from build123d import *

# Parameters (mm, degrees)
SKETCH_1_W               = 55
SKETCH_1_H               = 55
EXTRUDE_1_DEPTH          = 4
FILLET_1_R               = 3.5
SKETCH_2_R               = 13.15
CUT_EXTRUDE_1_DEPTH      = 4
SKETCH_3_R               = 2.1
CUT_EXTRUDE_2_DEPTH      = 4
PATTERN_CIRCULAR_1_COUNT = 4
CUT_EXTRUDE_3_DEPTH      = 4
PATTERN_CIRCULAR_2_COUNT = 4


with BuildPart() as part:
    # 草图1 → 凸台-拉伸1 (new body)
    with BuildSketch(Plane(origin=(0, 0, 0), x_dir=(1, 0, 0), z_dir=(0, 1, 0))):
        Rectangle(SKETCH_1_W, SKETCH_1_H)
    extrude(amount=EXTRUDE_1_DEPTH)

    # 圆角1
    fillet_1_edges = [part.edges().sort_by_distance(p)[0] for p in [
        (27.5, 2, 27.5),
        (-27.5, 2, 27.5),
        (-27.5, 2, -27.5),
        (27.5, 2, -27.5),
    ]]
    fillet(fillet_1_edges, radius=FILLET_1_R)

    # 草图2 → 切除-拉伸1 (cut)
    with BuildSketch(Plane(origin=(0, 4, 0), x_dir=(1, 0, 0), z_dir=(0, 1, 0))):
        with Locations(Location((0, 0, 0), (0, 0, 270))):
            Circle(SKETCH_2_R)
    extrude(amount=-CUT_EXTRUDE_1_DEPTH, mode=Mode.SUBTRACT)

    # 草图3 → 切除-拉伸2 (cut)
    with BuildSketch(Plane(origin=(0, 4, 0), x_dir=(1, 0, 0), z_dir=(0, 1, 0))):
        with Locations(Location((0, 17.5, 0), (0, 0, 270))):
            Circle(SKETCH_3_R)
    cut_extrude_2 = extrude(amount=-CUT_EXTRUDE_2_DEPTH, mode=Mode.SUBTRACT)

    # 阵列(圆周)1: 切除-拉伸2 ×4 about axis
    pattern_circular_1_axis = Axis((0, 0, 0), (0, 1, 0))
    for i in range(1, PATTERN_CIRCULAR_1_COUNT):
        add(cut_extrude_2.rotate(pattern_circular_1_axis, i * 360 / PATTERN_CIRCULAR_1_COUNT), mode=Mode.SUBTRACT)

    # 草图4 → 切除-拉伸3 (cut)
    with BuildSketch(Plane(origin=(0, 4, 0), x_dir=(1, 0, 0), z_dir=(0, 1, 0))):
        with BuildLine():
            ThreePointArc((-21.9, 24), (-25.48492424, 25.48492424), (-24, 21.9))
            Line((-24, 21.9), (-24, 24))
            Line((-24, 24), (-21.9, 24))
        make_face()
        with BuildLine():
            Line((-24, 24), (-24, 21.9))
            ThreePointArc((-24, 21.9), (-22.51507576, 22.51507576), (-21.9, 24))
            Line((-21.9, 24), (-24, 24))
        make_face()
    cut_extrude_3 = extrude(amount=-CUT_EXTRUDE_3_DEPTH, mode=Mode.SUBTRACT)

    # 阵列(圆周)2: 切除-拉伸3 ×4 about axis
    pattern_circular_2_axis = Axis((0, 0, 0), (0, 1, 0))
    for i in range(1, PATTERN_CIRCULAR_2_COUNT):
        add(cut_extrude_3.rotate(pattern_circular_2_axis, i * 360 / PATTERN_CIRCULAR_2_COUNT), mode=Mode.SUBTRACT)


solid = part.part
Check sheet for the modelled part. Datum: model origin and axes. Units: mm. Round coordinates to 2 decimals unless told otherwise and drop trailing zeros. Order: outer loops, then holes, each group sorted by start corner. A loop starts at its lowest first (then second) coordinate and runs counter-clockwise, first axis right, second up.
Q1. Cross-section at C-C, the plane y = 2.8. Give the number of separate pieces and of enclosed holes in the cut face, plus the area to 3 significant figures.
Filled sheet:
separate pieces: 1
enclosed holes: 9
area: 2,360 mm2
Q2. Scan lines: L1, parallel to X at y = 1.3, z = -17.5; L2, parallel to Z at x = 22.5, y = 0.35; L3, parallel to Z at x = 23, y = 0.8. Record each from-to range of solid material in increasing order.
Filled sheet:
L1: x = -27.5 to -2.1, 2.1 to 27.5
L2: z = -27.5 to -25.47, -22.53 to 22.53, 25.47 to 27.5
L3: z = -27.5 to -25.85, -22.15 to 22.15, 25.85 to 27.5
Q3. Cross-section at D-D, the plane x = 0. Enter the section's corners in (y, z), plus the area to 3 significant figures.
Filled sheet:
outline: (0, -27.5) - (4, -27.5) - (4, -19.6) - (0, -19.6) - close; (0, -15.4) - (4, -15.4) - (4, -13.15) - (0, -13.15) - close; (0, 13.15) - (4, 13.15) - (4, 15.4) - (0, 15.4) - close; (0, 19.6) - (4, 19.6) - (4, 27.5) - (0, 27.5) - close
area: 81.2 mm2
Q4. Cross-section at B-B, the plane x = -17.5. Enter the section's corners in (y, z).
Filled sheet:
outline: (0, -27.5) - (4, -27.5) - (4, -2.1) - (0, -2.1) - close; (0, 2.1) - (4, 2.1) - (4, 27.5) - (0, 27.5) - close
Q5. Draft check along Z on faces 1 (the face through (15.497, 2.028, 0.631)), 2 (the face through (-26.5, 2.03, 26.45)), 3 (the face through (-13, 4, -6)). Enter one of: pulls with the +Z half, pulls with the -Z half, needs draft (parallel to the pull), parting line crosses it, or undercut.
Filled sheet:
face 1: undercut
face 2: pulls with the +Z half
face 3: needs draft
Q6. Cross-section at A-A, the plane z = 0. Enter the section's corners in (x, y).
Filled sheet:
outline: (-27.5, 0) - (-19.6, 0) - (-19.6, 4) - (-27.5, 4) - close; (-15.4, 0) - (-13.15, 0) - (-13.15, 4) - (-15.4, 4) - close; (13.15, 0) - (15.4, 0) - (15.4, 4) - (13.15, 4) - close; (19.6, 0) - (27.5, 0) - (27.5, 4) - (19.6, 4) - close
Q7. Depth check by flat-ended pin: P1, Ø4, axis at x = 3, z = 9, coming from the +Y side. Enter the tip coordinate at first touch or a pass-through.
Filled sheet:
P1: passes through
